Verification items for this drawing (mm, ordinates from the low corner). A direction names the side the tool comes from. Round coordinates to 2 decimals unless told otherwise and drop trailing zeros. Write each loop counter-clockwise with the first axis right and the second up, starting at its lowest first coordinate (ties: lowest second). Pieces come first, ordered by that corner, then holes. Notation, with made-up numbers: M 41.25,65.25 L 53.25,65.25 A33 cw 53.25,104.25 Z; hole C 78,0 d4. An arc over 180 degrees is marked long. Write each question's results on one line, items separated by ' | '.
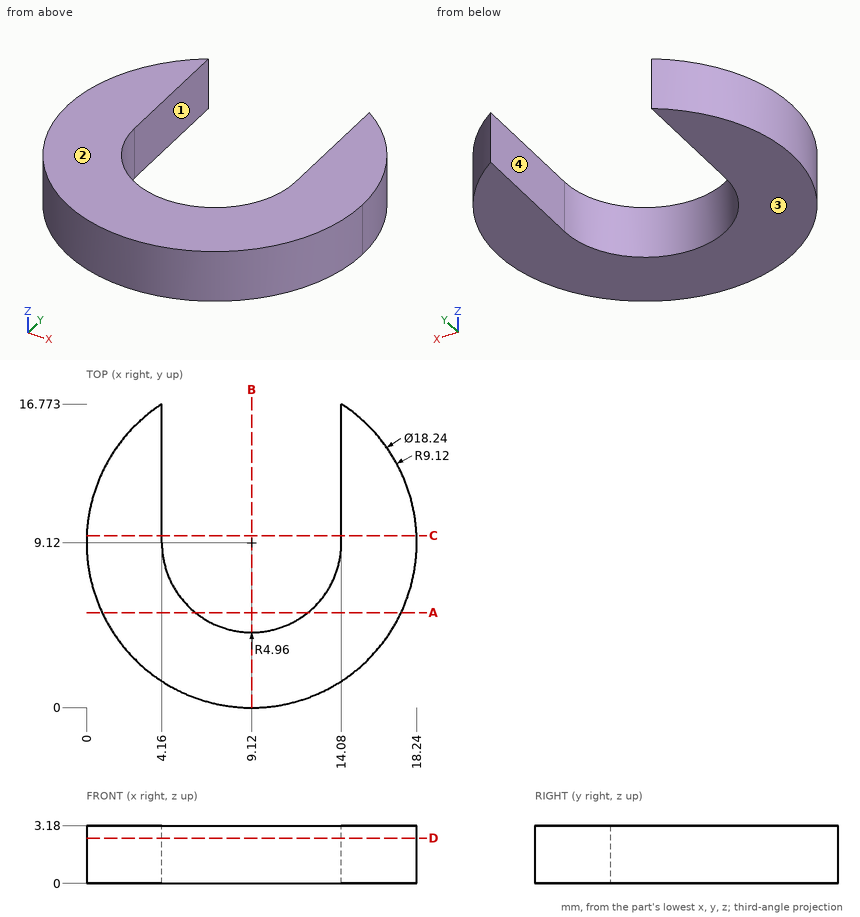
1) Sectioned sample at C-C, the plane y = 9.5. Record the cut outline in (x, z), and give its area (3 significant figures).
Calculated:
outline: M 0.01,0 L 4.16,0 L 4.16,3.18 L 0.01,3.18 Z; M 14.08,0 L 18.23,0 L 18.23,3.18 L 14.08,3.18 Z | area: 26.4 mm²
2) Depth check by flat-ended pin: P1, Ø1.6, axis at y = 14, z = 1, coming from the -X side; P2, Ø1.5, axis at x = 11.5, z = 1, coming from the +Y side; P3, Ø1, axis at y = 13.5, z = 2.5, coming from the +X side. Enter the tip coordinate at first touch or a pass-through.
Calculated:
P1: stops at x = 0.96 | P2: stops at y = 5.27 | P3: stops at x = 17.37
3) Access from +Z, -Z, +X, -X, +Y, -Y to the whole of each face (thin tool, end or side, straight path). Record for the marked faces 1 and 2.
Calculated:
face 1: +Z, -Z, +Y | face 2: +Z, +X, -X, +Y, -Y
4) Material ranges on line 1 (X direction, y = 7.5, z = 1.6) (1 decimal); line 2 (X direction, y = 7.25, z = 1.95) (1 decimal); line 3 (Y direction, x = 13.5, z = 1.05) (1 decimal), recorded low to high. Write a range as [from, to].
Calculated:
line 1: x = [0.1, 4.4], [13.8, 18.1] | line 2: x = [0.2, 4.5], [13.7, 18] | line 3: y = [1.1, 6.8]
5) Sectioned sample at B-B, the plane x = 9.12. Record the cut outline in (y, z), and give its area (3 significant figures).
Calculated:
outline: M 0,0 L 4.16,0 L 4.16,3.18 L 0,3.18 Z | area: 13.2 mm²
6) Sectioned sample at A-A, the plane y = 5.25. Record the cut outline in (x, z).
Calculated:
outline: M 0.86,0 L 6.02,0 L 6.02,3.18 L 0.86,3.18 Z; M 12.22,0 L 17.38,0 L 17.38,3.18 L 12.22,3.18 Z
7) Sectioned sample at D-D, the plane z = 2.5. Record the cut outline in (x, y).
Calculated:
outline: M 4.16,9.12 L 4.16,16.77 A9.12 ccw long 14.08,16.77 L 14.08,9.12 A4.96 cw Z
8) Draft check along X on the marked faces 3 and 4. Enter one of: pulls with the +X half, pulls with the -X half, needs draft (parallel to the pull), parting line crosses it, or undercut.
Calculated:
face 3: needs draft | face 4: undercut
